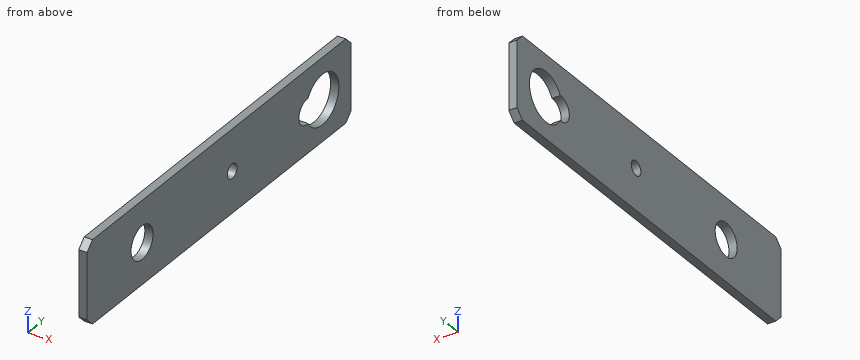
from build123d import *

# Parameters (mm, degrees)
SKETCH1_W           = 20
SKETCH1_H           = 96
BOSS_EXTRUDE1_DEPTH = 2
SKETCH2_R           = 1.75
SKETCH2_R_2         = 4
CUT_EXTRUDE1_DEPTH  = 99.081598682
CHAMFER1_SIZE       = 2


with BuildPart() as part:
    # Sketch1 → Boss-Extrude1 (new body)
    with BuildSketch(Plane(origin=(0, 0, 0), x_dir=(0, 0, -1), z_dir=(1, 0, 0))):
        with Locations((10, 48)):
            Rectangle(SKETCH1_W, SKETCH1_H)
    extrude(amount=BOSS_EXTRUDE1_DEPTH)

    # Sketch2 → Cut-Extrude1 (cut, through all)
    with BuildSketch(Plane(origin=(2, 0, 0), x_dir=(0, 0, -1), z_dir=(1, 0, 0))):
        with Locations((10, 52.75)):
            Circle(SKETCH2_R)
        with Locations((10, 20)):
            Circle(SKETCH2_R_2)
        with BuildLine():
            ThreePointArc((12.985415651, 80.295454545), (10, 91.5), (7.014584349, 80.295454545))
            ThreePointArc((7.014584349, 80.295454545), (10, 77), (12.985415651, 80.295454545))
        make_face()
    extrude(amount=-CUT_EXTRUDE1_DEPTH, mode=Mode.SUBTRACT)

    # Chamfer1
    chamfer1_edges = [part.edges().sort_by_distance(p)[0] for p in [
        (1, 96, 0),
        (1, 96, -20),
        (1, 0, -20),
        (1, 0, 0),
    ]]
    chamfer(chamfer1_edges, length=CHAMFER1_SIZE)


solid = part.part
Verification items for the finished model (mm, model axes). Give positions to 0.01 mm unless a question says otherwise; leave off trailing zeros. Loops run counter-clockwise (first coordinate to the right, second up) from the corner with the lowest first, then second, coordinate; pieces in that order, holes last.
1) Thickness scan on line 1 along Z through (x, y) = (1.5, 85.5); line 2 along Z through (x, y) = (0.7, 80); line 3 along Y through (x, z) = (0.5, -9). Record the ranges inside material, lowest first.
2) Sectioned sample at B-B, the plane z = -10. Enter the section's corners in (x, y).
3) Sectioned sample at D-D, the plane y = 52.75. Enter the section's corners in (x, z).
4) Sectioned sample at A-A, the plane y = 20. Enter the section's corners in (x, z), then the cut area to 3 significant figures.
5) Sectioned sample at C-C, the plane x = 1.4. Enter the section's corners in (y, z).
Answers:
1. line 1: z = -20 to -16, -4 to 0
1. line 2: z = -20 to -13, -7 to 0
1. line 3: y = 0 to 16.13, 23.87 to 51.31, 54.19 to 77.17, 91.42 to 96
2. outline: (0, 0) - (2, 0) - (2, 16) - (0, 16) - close; (0, 24) - (2, 24) - (2, 51) - (0, 51) - close; (0, 54.5) - (2, 54.5) - (2, 77) - (0, 77) - close; (0, 91.5) - (2, 91.5) - (2, 96) - (0, 96) - close
3. outline: (0, -20) - (2, -20) - (2, -11.75) - (0, -11.75) - close; (0, -8.25) - (2, -8.25) - (2, 0) - (0, 0) - close
4. outline: (0, -20) - (2, -20) - (2, -14) - (0, -14) - close; (0, -6) - (2, -6) - (2, 0) - (0, 0) - close
4. area: 24.0 mm2
5. outline: (0, -18) - (2, -20) - (94, -20) - (96, -18) - (96, -2) - (94, 0) - (2, 0) - (0, -2) - close; hole circle Ø8 at (20, -10); hole circle Ø3.5 at (52.75, -10); hole (80.3, -12.99) arc R6 ccw (long way) to (80.3, -7.01) arc R3 ccw (long way) to start
